```python
from build123d import *

# Parameters (mm, degrees)
F0_W     = 127
F0_H     = 107.95
F1_DEPTH = 25.4
F2_W     = 25.4
F2_H     = 19.05
F3_DEPTH = 12.7
F4_R     = 3.175
F5_R     = 1.524
F6_R     = 12.7
F7_R     = 3.175


with BuildPart() as f1:
    # F0 (on Top) → F1 (new body)
    with BuildSketch(Plane.XY):
        Rectangle(F0_W, F0_H)
    extrude(amount=F1_DEPTH)

    # F2 (on face) → F3 (cut)
    with BuildSketch(Plane.XY.offset(25.4)):
        with Locations((-38.1, 31.75)):
            Rectangle(F2_W, F2_H)
    extrude(amount=-F3_DEPTH, mode=Mode.SUBTRACT)

    # F4
    f4_edges = [f1.edges().sort_by_distance(p)[0] for p in [
        (-50.8, 41.275, 19.05),
        (-50.8, 22.225, 19.05),
        (-25.4, 22.225, 19.05),
        (-25.4, 41.275, 19.05),
    ]]
    fillet(f4_edges, radius=F4_R)

    # F5
    f5_edges = [f1.edges().sort_by_distance(p)[0] for p in [
        (-38.1, 22.225, 12.7),
    ]]
    fillet(f5_edges, radius=F5_R)

    # F6
    f6_edges = [f1.edges().sort_by_distance(p)[0] for p in [
        (63.5, -53.975, 12.7),
        (63.5, 53.975, 12.7),
        (-63.5, -53.975, 12.7),
        (-63.5, 53.975, 12.7),
    ]]
    fillet(f6_edges, radius=F6_R)

    # F7
    f7_edges = [f1.edges().sort_by_distance(p)[0] for p in [
        (0, -53.975, 25.4),
    ]]
    fillet(f7_edges, radius=F7_R)


solid = f1.part
```
Work out the finished part from the listing and answer in its coordinate system (mm). A direction names the side the tool comes from. Round coordinates to 2 decimals unless told otherwise and drop trailing zeros. Loops run counter-clockwise (first coordinate to the right, second up) from the corner with the lowest first, then second, coordinate; pieces in that order, holes last.
(1) The part is cut by section A-A, the plane z = 20.75. Give the vertices of the cut face in (x, y) (3 decimals).
Computed values:
outline: (-63.5, -41.275) arc R12.7 ccw to (-50.8, -53.975) - (50.8, -53.975) arc R12.7 ccw to (63.5, -41.275) - (63.5, 41.275) arc R12.7 ccw to (50.8, 53.975) - (-50.8, 53.975) arc R12.7 ccw to (-63.5, 41.275) - close; hole (-50.8, 25.4) arc R3.175 ccw to (-47.625, 22.225) - (-28.575, 22.225) arc R3.175 ccw to (-25.4, 25.4) - (-25.4, 38.1) arc R3.175 ccw to (-28.575, 41.275) - (-47.625, 41.275) arc R3.175 ccw to (-50.8, 38.1) - close
(2) Find the intervals of material crossed by L1, parallel to X at y = 34, z = 22.5; L2, parallel to Y at x = -49, z = 23; L3, parallel to X at y = -39, z = 23.25, in increasing order.
Computed values:
L1: x = -63.49 to -50.8, -25.4 to 63.49
L2: y = -53.88 to 22.54, 40.96 to 53.88
L3: x = -63.33 to 63.33
(3) This flat-tipped pin is pushed along its axis until it touches: P1, Ø5, axis at x = -38, y = 29.5, coming from the +Z side. Where does it stop, or does it pass through?
Computed values:
P1: stops at z = 12.7
(4) The mould has two halves that part along X. Classify faces 1 (the cylindrical face through (-59.878, -50.156, 11.268)), 2 (the cylindrical face through (62.55, 0.58, 24.49)), 3 (the cylindrical face through (-26.305, 40.32, 19.734)), 4 (the cylindrical face through (-49.845, 40.37, 19.734)): pulls with the +X half, pulls with the -X half, needs draft (parallel to the pull), parting line crosses it, or undercut.
Computed values:
face 1: pulls with the -X half
face 2: pulls with the +X half
face 3: undercut
face 4: undercut
(5) For faces 5 (the cylindrical face through (-26.355, 23.13, 19.734)), 6 (the flat face through (-1, 1, 25.4)), determine the directions among +Z, -Z, +X, -X, +Y, -Y from which every point of the face is accessible in a straight line to the end or side of a thin tool.
Computed values:
face 5: +Z
face 6: +Z, +X, -X, +Y, -Y
(6) The part is cut by section B-B, the plane y = 35.5. Give the vertices of the cut face in (x, z) (3 decimals).
Computed values:
outline: (-63.5, 0) - (63.5, 0) - (63.5, 22.225) arc R3.175 ccw to (60.325, 25.4) - (-25.4, 25.4) - (-25.4, 14.224) arc R1.524 cw to (-26.924, 12.7) - (-49.276, 12.7) arc R1.524 cw to (-50.8, 14.224) - (-50.8, 25.4) - (-60.325, 25.4) arc R3.175 ccw to (-63.5, 22.225) - close
